Could you check a few things on this drawing? It's one solid part, dimensions in mm from its lowest x, y, z. Round coordinates to 2 decimals unless told otherwise and drop trailing zeros. Order: outer loops, then holes, each group sorted by start corner. A loop starts at its lowest first (then second) coordinate and runs counter-clockwise, first axis right, second up.
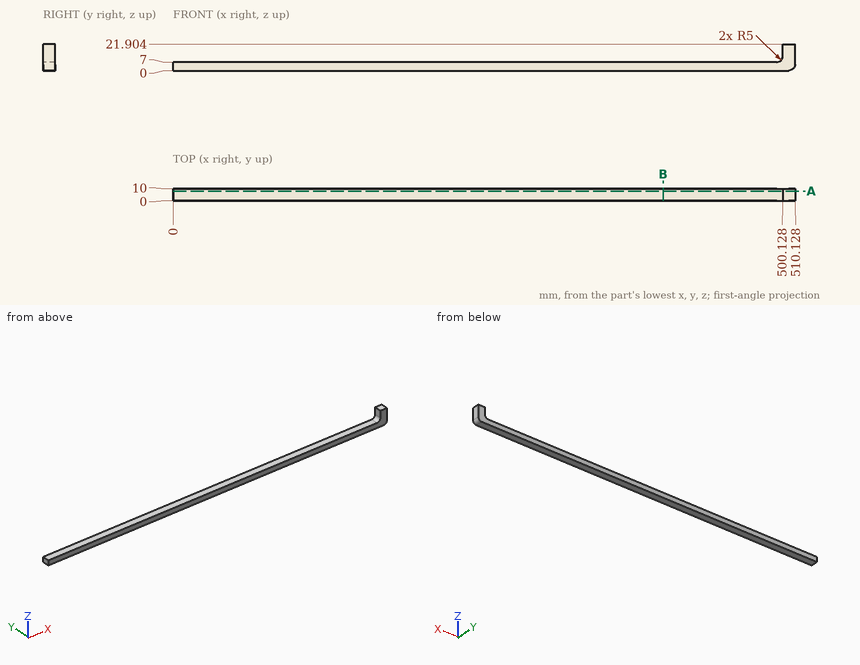
(1) Please list where these lines run through material, in increasing order: probe 1 along X at (y, z) = (4.25, 18); probe 2 along Z at (x, y) = (283, 8.5); probe 3 along X at (y, z) = (5.25, 9.75).
(2) I want a section at A-A, the plane y = 8. List the corners of the cut face in (x, z) for me (1 decimal).
(3) I want a section at B-B, the plane x = 402. List the corners of the cut face in (y, z) for me.
(4) I'm going to push flat-ended pins straight in: pin 1 Ø3 at (x, y) = (134, 7) entering from +Z; pin 2 Ø3 at (y, z) = (8, 19.5) entering from -X. Where does each tip first touch, or does it pass through?
Ans:
1. probe 1: x = 500.13 to 510.13
1. probe 2: z = 0 to 7
1. probe 3: x = 499.59 to 510.13
2. outline: (0, 0) - (505.1, 0) arc R5 ccw to (510.1, 5) - (510.1, 21.9) - (500.1, 21.9) - (500.1, 12) arc R5 cw to (495.1, 7) - (0, 7) - close
3. outline: (0, 0) - (10, 0) - (10, 7) - (0, 7) - close
4. pin 1: stops at z = 7
4. pin 2: stops at x = 500.13
